Verification items for the finished model (mm, model axes). Coordinates: 2 decimals unless noted, no trailing zeros. Loops run counter-clockwise (first coordinate to the right, second up) from the corner with the lowest first, then second, coordinate; pieces in that order, holes last.
Q1. Sectioned sample at D-D (x = 54). Enter the section's corners in (y, z), then the cut area to 3 significant figures.
Q2. Sectioned sample at B-B (x = 23). Enter the section's corners in (y, z).
Q3. Go/stop test with flat-tipped pins: P1, Ø2.5, axis at x = 23.25, y = -48.3, coming from the -Z side; P2, Ø0.9, axis at y = -44, z = 1.5, coming from the -X side; P3, Ø1.5, axis at x = 24, z = 1.5, coming from the +Y side. Record where each tip stops, or that it passes through.
Q4. Material ranges on probe 1 along Y at (x, z) = (20, 0.9); probe 2 along Y at (x, z) = (8.5, 1.95); probe 3 along Y at (x, z) = (24, 1.9), recorded low to high.
Q5. Sectioned sample at A-A (x = 14.5). Enter the section's corners in (y, z), then the cut area to 3 significant figures.
Q6. Sectioned sample at C-C (z = 1.2). Enter the section's corners in (x, y).
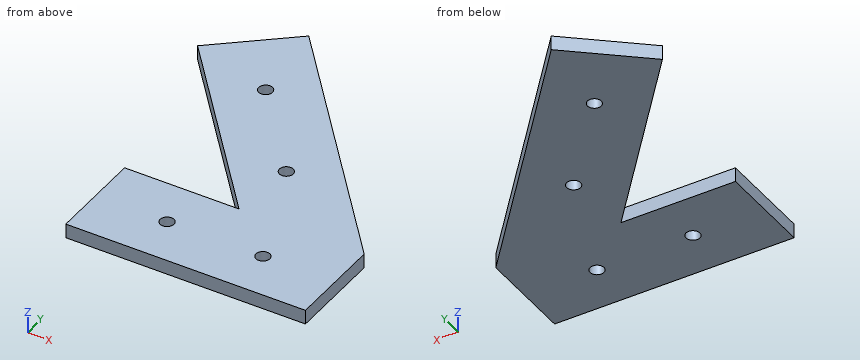
```python
from build123d import *

# Parameters (mm, degrees)
SKETCH1_R           = 1.45
BOSS_EXTRUDE1_DEPTH = 3


with BuildPart() as part:
    # Sketch1 → Boss-Extrude1 (new body)
    with BuildSketch(Plane.XY):
        Polygon((0, 0), (32.139380484, -38.302222156), (8.247526271, -38.302222156), (8.247526271, -58.302222156), (58.247526271, -58.302222156), (58.247526271, -38.302222156), (15.320888862, 12.855752194), align=None)
        with Locations((23.247526271, -48.302222156)):
            Circle(SKETCH1_R, mode=Mode.SUBTRACT)
        with Locations((43.247526271, -48.302222156)):
            Circle(SKETCH1_R, mode=Mode.SUBTRACT)
        with Locations((17.302258576, -5.06279055)):
            Circle(SKETCH1_R, mode=Mode.SUBTRACT)
        with Locations((33.371948819, -24.213901628)):
            Circle(SKETCH1_R, mode=Mode.SUBTRACT)
    extrude(amount=BOSS_EXTRUDE1_DEPTH)


solid = part.part
```
Geometry check:
1. outline: (-58.3, 0) - (-33.24, 0) - (-33.24, 3) - (-58.3, 3) - close
1. area: 75.2 mm2
2. outline: (-58.3, 0) - (-49.73, 0) - (-49.73, 3) - (-58.3, 3) - close; (-46.87, 0) - (-38.3, 0) - (-38.3, 3) - (-46.87, 3) - close; (-27.41, 0) - (3.7, 0) - (3.7, 3) - (-27.41, 3) - close
3. P1: passes through
3. P2: stops at x = 8.25
3. P3: stops at y = 3.41
4. probe 1: y = -58.3 to -38.3, -23.84 to 7.28
4. probe 2: y = -58.3 to -38.3, -10.13 to 7.13
4. probe 3: y = -58.3 to -49.54, -47.06 to -38.3, -28.6 to 2.51
5. outline: (-58.3, 0) - (-38.3, 0) - (-38.3, 3) - (-58.3, 3) - close; (-17.28, 0) - (12.17, 0) - (12.17, 3) - (-17.28, 3) - close
5. area: 148 mm2
6. outline: (0, 0) - (32.14, -38.3) - (8.25, -38.3) - (8.25, -58.3) - (58.25, -58.3) - (58.25, -38.3) - (15.32, 12.86) - close; hole circle Ø2.9 at (17.3, -5.06); hole circle Ø2.9 at (23.25, -48.3); hole circle Ø2.9 at (33.37, -24.21); hole circle Ø2.9 at (43.25, -48.3)
